Print and shaded views of the part. All mm, measured from the part's lowest x, y and z. Give positions to 0.01 mm unless a question says otherwise; leave off trailing zeros. Loops run counter-clockwise (first coordinate to the right, second up) from the corner with the lowest first, then second, coordinate; pieces in that order, holes last. Notation, with made-up numbers: M 11.5,59 L 63.5,59 A16 cw 63.5,87 Z; hole C -9,67.25 d8. An arc over 180 degrees is marked long. Answer in a Markdown table with one row per item.
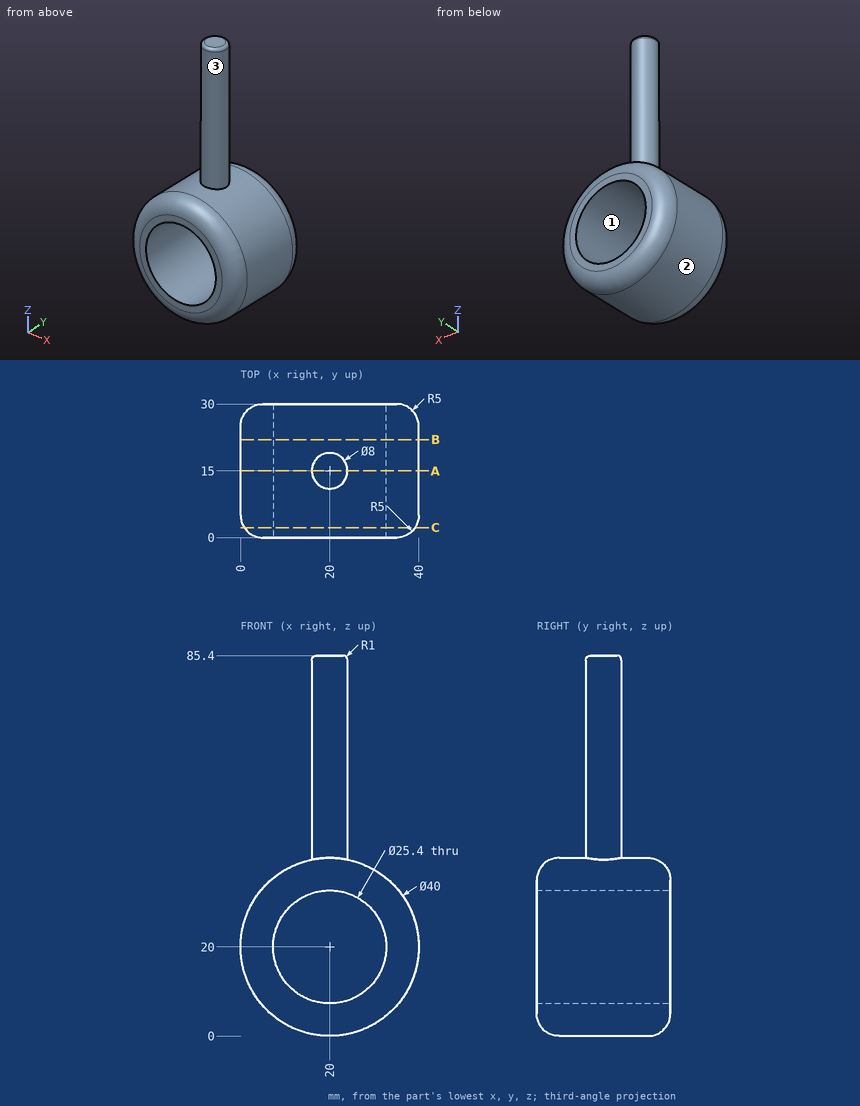
(1) Saw through at B-B, the plane y = 22. Give the cut face in (x, z), and give its area (3 significant figures).
Established:
| item | result |
|---|---|
| outline | C 20,20 d40; hole C 20,20 d25.4 |
| area | 750 mm2 |
(2) Flat gauge pins, fed straight in: P1, Ø4, axis at x = 28, y = 22.5, coming from the -Z side; P2, Ø5, axis at x = 34.5, y = 11.5, coming from the +Z side; P3, Ø5, axis at x = 20, y = 16, coming from the -Z side. Where does each tip first touch, or does it go through?
Established:
| item | result |
|---|---|
| P1 | stops at z = 0.92 |
| P2 | stops at z = 36 |
| P3 | stops at z = 0 |
(3) Wall check: L1, parallel to Z at x = 20, y = 10.75; L2, parallel to Z at x = 20, y = 15.5; L3, parallel to Y at x = 18.5, z = 40.5. Give the ranges that are in metal, low to high.
Established:
| item | result |
|---|---|
| L1 | z = 0 to 7.3, 32.7 to 40 |
| L2 | z = 0 to 7.3, 32.7 to 85.4 |
| L3 | y = 11.29 to 18.71 |
(4) Saw through at C-C, the plane y = 2.25. Give the cut face in (x, z).
Established:
| item | result |
|---|---|
| outline | C 20,20 d38.35; hole C 20,20 d25.4 |
(5) Mould opens along Z. For the marked faces 1, 2 and 3 say: pulls with the +Z half, pulls with the -Z half, needs draft (parallel to the pull), parting line crosses it, or undercut.
Established:
| item | result |
|---|---|
| face 1 | undercut |
| face 2 | parting line crosses it |
| face 3 | needs draft |
(6) Saw through at A-A, the plane y = 15. Give the cut face in (x, z), and give its area (3 significant figures).
Established:
| item | result |
|---|---|
| outline | M 16,39.6 A20 ccw long 24,39.6 L 24,84.4 A1 ccw 23,85.4 L 17,85.4 A1 ccw 16,84.4 Z; hole C 20,20 d25.4 |
| area | 1,110 mm2 |
